Can you work these out from the model? Positions are in its coordinate system, mm. A direction names the side the tool comes from. Give positions to 0.01 mm unless a question says otherwise; leave off trailing zeros. Write each loop counter-clockwise with the first axis right and the second up, starting at its lowest first coordinate (ties: lowest second). Pieces come first, ordered by that corner, then holes.
```python
from build123d import *

# Parameters (mm, degrees)
SKETCH1_W               = 150
SKETCH1_H               = 170
BOSS_EXTRUDE1_DEPTH     = 62.5
CUT_EXTRUDE1_DEPTH      = 197.038899201
CUT_EXTRUDE1_DEPTH_BACK = 197.038899201
CUT_EXTRUDE2_START      = -4
CUT_EXTRUDE2_DEPTH      = 180.388249351
SKETCH4_R               = 2.5
CUT_EXTRUDE3_DEPTH      = 181.131202346
SKETCH7_W               = 38.956320025
SKETCH7_H               = 38.29066934
SKETCH7_R               = 12.51992823
CUT_EXTRUDE4_DEPTH      = 5


with BuildPart() as part:
    # Sketch1 → Boss-Extrude1 (new, symmetric)
    with BuildSketch(Plane(origin=(0, 0, 0), x_dir=(0, 0, -1), z_dir=(1, 0, 0))):
        Rectangle(SKETCH1_W, SKETCH1_H)
    extrude(amount=BOSS_EXTRUDE1_DEPTH, both=True)

    # Sketch2 → Cut-Extrude1 (cut, two sides: drawn at the far end of the back side and taken through both)
    with BuildSketch(Plane(origin=(0, 85, 0), x_dir=(1, 0, 0), z_dir=(0, 1, 0)).offset(-CUT_EXTRUDE1_DEPTH_BACK)):
        with BuildLine():
            Line((-399.296963127, -111.543444717), (-62.5, 60))
            ThreePointArc((-62.5, 60), (0, 75), (62.5, 60))
            Line((62.5, 60), (399.296963127, -111.543444717))
            Line((399.296963127, -111.543444717), (399.296963127, 644.391335002))
            Line((399.296963127, 644.391335002), (-399.296963127, 644.391335002))
            Line((-399.296963127, 644.391335002), (-399.296963127, -111.543444717))
        make_face()
    extrude(amount=CUT_EXTRUDE1_DEPTH + CUT_EXTRUDE1_DEPTH_BACK, mode=Mode.SUBTRACT)

    # Sketch3 → Cut-Extrude2 (cut, through all)
    with BuildSketch(Plane.XY.offset(75).offset(CUT_EXTRUDE2_START)):
        with BuildLine():
            Line((50.5, 125.138194242), (106.621589134, 125.138194242))
            Line((106.621589134, 125.138194242), (106.621589134, 73))
            Line((106.621589134, 73), (53.5, 73))
            ThreePointArc((53.5, 73), (51.378679656, 73.878679656), (50.5, 76))
            Line((50.5, 76), (50.5, 125.138194242))
        make_face()
        with BuildLine():
            Line((-106.621589134, 125.138194242), (-106.621589134, 73))
            Line((-106.621589134, 73), (-53.5, 73))
            ThreePointArc((-53.5, 73), (-51.378679656, 73.878679656), (-50.5, 76))
            Line((-50.5, 76), (-50.5, 125.138194242))
            Line((-50.5, 125.138194242), (-106.621589134, 125.138194242))
        make_face()
        with BuildLine():
            Line((-50.5, -125.138194242), (-106.621589134, -125.138194242))
            Line((-106.621589134, -125.138194242), (-106.621589134, -73))
            Line((-106.621589134, -73), (-53.5, -73))
            ThreePointArc((-53.5, -73), (-51.378679656, -73.878679656), (-50.5, -76))
            Line((-50.5, -76), (-50.5, -125.138194242))
        make_face()
        with BuildLine():
            Line((106.621589134, -125.138194242), (106.621589134, -73))
            Line((106.621589134, -73), (53.5, -73))
            ThreePointArc((53.5, -73), (51.378679656, -73.878679656), (50.5, -76))
            Line((50.5, -76), (50.5, -125.138194242))
            Line((50.5, -125.138194242), (106.621589134, -125.138194242))
        make_face()
    extrude(amount=-CUT_EXTRUDE2_DEPTH, mode=Mode.SUBTRACT)

    # Sketch4 → Cut-Extrude3 (cut, through all)
    with BuildSketch(Plane(origin=(0, 0, 71), x_dir=(-1, 0, 0), z_dir=(0, 0, -1))):
        with Locations((-56.75, 77.5)):
            Circle(SKETCH4_R)
        with Locations(Location((56.75, 77.5, 0), (0, 0, 180))):
            Circle(SKETCH4_R)
        with Locations((56.75, -77.5)):
            Circle(SKETCH4_R)
        with Locations(Location((-56.75, -77.5, 0), (0, 0, 180))):
            Circle(SKETCH4_R)
    extrude(amount=-CUT_EXTRUDE3_DEPTH, mode=Mode.SUBTRACT)

    # Sketch7 → Cut-Extrude4 (cut)
    with BuildSketch(Plane(origin=(0, 85, 0), x_dir=(1, 0, 0), z_dir=(0, 1, 0))):
        with Locations((-15.997309365, -55.85466533)):
            Rectangle(SKETCH7_W, SKETCH7_H)
        with Locations(Location((-15.997309365, -55.85466533, 0), (0, 0, 270))):
            Circle(SKETCH7_R, mode=Mode.SUBTRACT)
    extrude(amount=-CUT_EXTRUDE4_DEPTH, mode=Mode.SUBTRACT)


solid = part.part
```
1) Suppose I cut it at A-A on x = 56.75. Write out the boundary of the cut face in (y, z), plus the area to 3 significant figures.
Values follow:
outline: (-85, 71) - (-80, 71) - (-80, 75) - (-85, 75) - close; (-75, 71) - (-73, 71) - (-73, -62.76) - (73, -62.76) - (73, 71) - (75, 71) - (75, 75) - (-75, 75) - close; (80, 71) - (85, 71) - (85, 75) - (80, 75) - close
area: 20,200 mm2
2) Please list where these lines run through material, in increasing order: L1, parallel to X at y = 77, z = 72; L2, parallel to Y at x = 56.75, z = 73.45; L3, parallel to Z at x = 0.5, y = 66.5.
Values follow:
L1: x = -62.5 to -59.2, -54.3 to 54.3, 59.2 to 62.5
L2: y = -85 to -80, -75 to 75, 80 to 85
L3: z = -75 to 75
3) For faces 4 (the face through (-58, -73, 4)), 5 (the face through (-7.536, 82.535, 46.627)), 6 (the face through (56.4, -80.2, 71)), which set-ups out of +Z, -Z, +X, -X, +Y, -Y let a thin tool reach every point of the face, with its end or its side?
Values follow:
face 4: -Z, -X, -Y
face 5: +Y
face 6: -Z, +X, -Y
4) For pin 1 Ø10 at (y, z) = (-79.5, 0) entering from +X; pin 2 Ø7 at (y, z) = (81, -27.5) entering from +X; pin 3 Ø4 at (x, y) = (-43.5, -12.5) entering from -Z, each with a flat end and sliding along its axis, tell me the tip position at first contact or that it passes through.
Values follow:
pin 1: stops at x = 50.9
pin 2: stops at x = 50.5
pin 3: stops at z = -68.6
5) Suppose I cut it at C-C on y = 66. Write out the boundary of the cut face in (x, z), plus the area to 3 significant figures.
Values follow:
outline: (-62.5, -60) arc R137.71 ccw to (62.5, -60) - (62.5, 75) - (-62.5, 75) - close
area: 18,100 mm2
6) Suppose I cut it at D-D on x = 37. Write out the boundary of the cut face in (y, z).
Values follow:
outline: (-85, -69.94) - (85, -69.94) - (85, 75) - (-85, 75) - close
7) Suppose I cut it at B-B on z = -32.5. Write out the boundary of the cut face in (x, y), plus the area to 3 significant figures.
Values follow:
outline: (-62.5, -73) - (-53.5, -73) arc R3 cw to (-50.5, -76) - (-50.5, -85) - (50.5, -85) - (50.5, -76) arc R3 cw to (53.5, -73) - (62.5, -73) - (62.5, 73) - (53.5, 73) arc R3 cw to (50.5, 76) - (50.5, 85) - (-50.5, 85) - (-50.5, 76) arc R3 cw to (-53.5, 73) - (-62.5, 73) - close
area: 20,700 mm2
8) If we mould it in two halves opening along X, with no side actions, what happens to faces 1 (the face through (-0.908, -1.19, -74.997)), 2 (the face through (1, 85, 1)), 3 (the face through (-16, 80, 43))? For each: +X half, -X half, draft (parallel to the pull), parting line (faces both ways), or undercut.
Values follow:
face 1: parting line
face 2: draft
face 3: undercut
